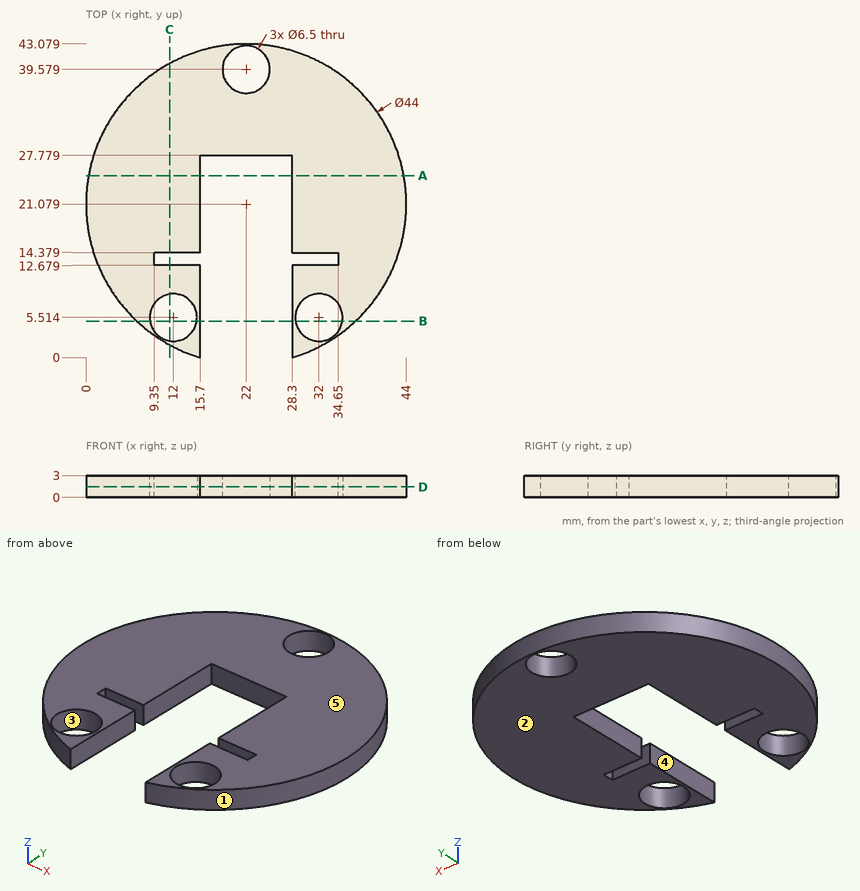
Design review of the part shown in the three views and the two pictorial views. Dimensions are in mm from the part's minimum x, y and z. A direction names the side the tool comes from. Give positions to 0.01 mm unless a question says otherwise; leave off trailing zeros. Write each loop counter-clockwise with the first axis right and the second up, starting at its lowest first coordinate (ties: lowest second). Pieces come first, ordered by that corner, then holes.
(1) Tool access review of the marked faces 4 and 5: name each direction out of +Z, -Z, +X, -X, +Y, -Y from which nothing blocks a thin tool from reaching the whole face with its end or side.
Checked values:
face 4: +Z, -Z, -Y
face 5: +Z, +X, -X, +Y, -Y
(2) Add section D-D (z = 1.45). Give the boundary of the cut face in (x, y).
Checked values:
outline: (9.35, 12.68) - (9.35, 14.38) - (15.7, 14.38) - (15.7, 27.78) - (28.3, 27.78) - (28.3, 14.38) - (34.65, 14.38) - (34.65, 12.68) - (28.3, 12.68) - (28.3, 0) arc R22 ccw (long way) to (15.7, 0) - (15.7, 12.68) - close; hole circle Ø6.5 at (12, 5.51); hole circle Ø6.5 at (22, 39.58); hole circle Ø6.5 at (32, 5.51)
(3) Add section A-A (y = 25). Give the boundary of the cut face in (x, z).
Checked values:
outline: (0.35, 0) - (15.7, 0) - (15.7, 3) - (0.35, 3) - close; (28.3, 0) - (43.65, 0) - (43.65, 3) - (28.3, 3) - close
(4) Add section C-C (x = 11.5). Give the boundary of the cut face in (y, z) (1 decimal).
Checked values:
outline: (1.7, 0) - (2.3, 0) - (2.3, 3) - (1.7, 3) - close; (8.7, 0) - (12.7, 0) - (12.7, 3) - (8.7, 3) - close; (14.4, 0) - (40.4, 0) - (40.4, 3) - (14.4, 3) - close
(5) Clearance check with flat-ended pins moving along their axes: pin 1 Ø1.4 at (y, z) = (13.5, 1) entering from +X; pin 2 Ø10 at (x, y) = (9.5, 38.5) entering from -Z; pin 3 Ø0.9 at (y, z) = (3, 2) entering from +X; pin 4 Ø1 at (x, z) = (36.5, 2) entering from +Y. State where each tip first meets the part, or that it passes through.
Checked values:
pin 1: stops at x = 42.9
pin 2: stops at z = 0
pin 3: stops at x = 35.16
pin 4: stops at y = 38.05
(6) Add section B-B (y = 5). Give the boundary of the cut face in (x, z), and give its area (3 significant figures).
Checked values:
outline: (6.98, 0) - (8.79, 0) - (8.79, 3) - (6.98, 3) - close; (15.21, 0) - (15.7, 0) - (15.7, 3) - (15.21, 3) - close; (28.3, 0) - (28.79, 0) - (28.79, 3) - (28.3, 3) - close; (35.21, 0) - (37.02, 0) - (37.02, 3) - (35.21, 3) - close
area: 13.8 mm2
(7) Wall thickness on line 1 along X through (y, z) = (7, 2.25) (1 decimal); line 2 along Y through (x, z) = (10.5, 0.1) (1 decimal); line 3 along Y through (x, z) = (10, 0.6) (1 decimal): over which ranges is each line inside the solid? List them lowest first.
Checked values:
line 1: x = 5.1 to 9.1, 14.9 to 15.7, 28.3 to 29.1, 34.9 to 38.9
line 2: y = 2.3 to 2.6, 8.4 to 12.7, 14.4 to 39.8
line 3: y = 2.6 to 3, 8.1 to 12.7, 14.4 to 39.5
(8) Mouldability with a two-part tool opening along Y and no side actions: class the marked faces 1, 2 and 3 as +Y half, -Y half, draft (parallel to the pull), parting line (faces both ways), or undercut.
Checked values:
face 1: parting line
face 2: draft
face 3: undercut
